from build123d import *

# Parameters (mm, degrees)
SKETCH1_W           = 10
SKETCH1_H           = 10
BOSS_EXTRUDE1_DEPTH = 10
SKETCH2_R           = 1
BOSS_EXTRUDE2_DEPTH = 2


with BuildPart() as part:
    # Sketch1 → Boss-Extrude1 (new body)
    with BuildSketch(Plane.XY):
        with Locations((5, -5)):
            Rectangle(SKETCH1_W, SKETCH1_H)
    extrude(amount=BOSS_EXTRUDE1_DEPTH)

    # Sketch2 → Boss-Extrude2 (add)
    with BuildSketch(Plane.XZ.offset(10)):
        with Locations(Location((5, 5, 0), (0, 0, 90))):
            Circle(SKETCH2_R)
    extrude(amount=BOSS_EXTRUDE2_DEPTH)


solid = part.part
Read the model definition and answer for the solid it produces. Units are mm, in the model's axes. A direction names the side the tool comes from. Round coordinates to 2 decimals unless told otherwise and drop trailing zeros. Write each loop counter-clockwise with the first axis right and the second up, starting at its lowest first coordinate (ties: lowest second). Pieces come first, ordered by that corner, then holes.
Q1. Find section C-C on z = 9.25. Determine the outline of the cut face in (x, y).
Values:
outline: (0, -10) - (10, -10) - (10, 0) - (0, 0) - close
Q2. A tool of negligible diameter and unlimited length cuts with its end or side. For faces 1 (the face through (5, -5, 0)), 2 (the face through (4, -11, 5)), from which of +Z, -Z, +X, -X, +Y, -Y can it reach the whole face along a straight path? Write none if from no direction.
Values:
face 1: -Z, +X, -X, +Y, -Y
face 2: -Y
Q3. Find section A-A on z = 5. Determine the outline of the cut face in (x, y).
Values:
outline: (0, -10) - (4, -10) - (4, -12) - (6, -12) - (6, -10) - (10, -10) - (10, 0) - (0, 0) - close
Q4. Straight lines are drawn through the part: line 1 (Y direction, x = 4, z = 3); line 2 (X direction, y = -10.5, z = 4.25). For each, find the intervals that lie inside material, in ascending order.
Values:
line 1: y = -10 to 0
line 2: x = 4.34 to 5.66
Q5. Find section B-B on x = 5. Determine the outline of the cut face in (y, z).
Values:
outline: (-12, 4) - (-10, 4) - (-10, 0) - (0, 0) - (0, 10) - (-10, 10) - (-10, 6) - (-12, 6) - close
Q6. Find section D-D on x = 1. Determine the outline of the cut face in (y, z).
Values:
outline: (-10, 0) - (0, 0) - (0, 10) - (-10, 10) - close
